```python
from build123d import *

# Parameters (mm, degrees)
ESQUISSE1_R             = 40
BOSS_EXTRU_1_DEPTH      = 78
ESQUISSE2_W             = 36.5
ESQUISSE2_H             = 3
ENL_V_MAT_EXTRU_1_DEPTH = 78
ESQUISSE3_R             = 3
ENL_V_MAT_EXTRU_2_DEPTH = 15


with BuildPart() as part:
    # Esquisse1 → Boss.-Extru.1 (new body)
    with BuildSketch(Plane.XY):
        with BuildLine():
            Line((-75, 0), (75, 0))
            Line((75, 0), (75, 15))
            Line((75, 15), (56.5, 15))
            Line((56.5, 15), (56.5, 83))
            Line((56.5, 83), (43.8178046, 83))
            ThreePointArc((43.8178046, 83), (0, 107), (-43.8178046, 83))
            Line((-43.8178046, 83), (-56.5, 83))
            Line((-56.5, 83), (-56.5, 15))
            Line((-56.5, 15), (-75, 15))
            Line((-75, 15), (-75, 0))
        make_face()
        with Locations((0, 55)):
            Circle(ESQUISSE1_R, mode=Mode.SUBTRACT)
    extrude(amount=BOSS_EXTRU_1_DEPTH)

    # Esquisse2 → Enlèv. mat.-Extru.1 (cut)
    with BuildSketch(Plane.XY.offset(78)):
        with Locations((38.25, 55)):
            Rectangle(ESQUISSE2_W, ESQUISSE2_H)
    extrude(amount=-ENL_V_MAT_EXTRU_1_DEPTH, mode=Mode.SUBTRACT)

    # Esquisse3 → Enlèv. mat.-Extru.2 (cut)
    with BuildSketch(Plane(origin=(0, 15, 0), x_dir=(1, 0, 0), z_dir=(0, 1, 0))):
        with Locations(Location((-65, -39, 0), (0, 0, 180))):
            Circle(ESQUISSE3_R)
        with Locations(Location((-65, -14, 0), (0, 0, 180))):
            Circle(ESQUISSE3_R)
        with Locations(Location((-65, -64, 0), (0, 0, 180))):
            Circle(ESQUISSE3_R)
        with Locations(Location((65, -64, 0), (0, 0, 180))):
            Circle(ESQUISSE3_R)
        with Locations(Location((65, -14, 0), (0, 0, 180))):
            Circle(ESQUISSE3_R)
        with Locations(Location((65, -39, 0), (0, 0, 180))):
            Circle(ESQUISSE3_R)
    extrude(amount=-ENL_V_MAT_EXTRU_2_DEPTH, mode=Mode.SUBTRACT)


solid = part.part
```
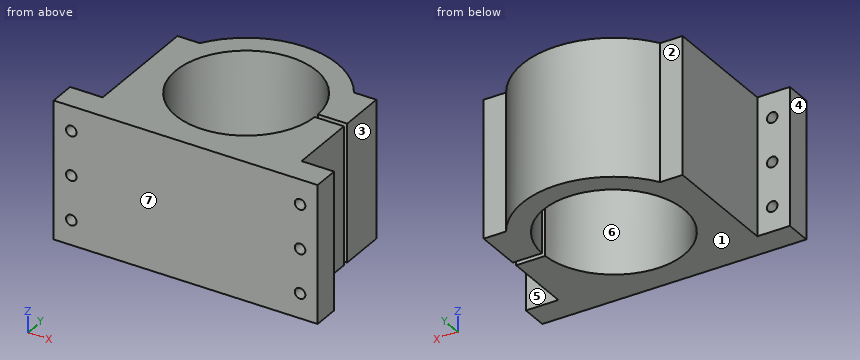
Geometry check sheet. Reference: the model listing, model coordinates, mm. Face numbers are marked on the shaded views. A direction names the side the tool comes from. Coordinates: 2 decimals unless noted, no trailing zeros. Write each loop counter-clockwise with the first axis right and the second up, starting at its lowest first coordinate (ties: lowest second). Pieces come first, ordered by that corner, then holes. Notation, with made-up numbers: M 1.5,35 L 38.5,35 A26 ccw 38.5,50 Z; hole C -13,8.5 d11. An arc over 180 degrees is marked long. Use one line per item in the form item = value. Start each with the question number.
1) Go/stop test with flat-tipped pins: pin 1 Ø9.5 at (x, z) = (-65, 14) entering from +Y; pin 2 Ø8 at (y, z) = (83.5, 34) entering from -X; pin 3 Ø20.5 at (x, z) = (66.5, 37) entering from +Y; pin 4 Ø5 at (x, z) = (65, 39) entering from +Y. Record where each tip stops, or that it passes through.
2) Thickness scan on probe 1 along Z at (x, y) = (65, 9); probe 2 along X at (y, z) = (12, 12); probe 3 along Y at (x, z) = (54, 8). Record the ranges inside material, lowest first. Write a range as from..to.
3) Set-up check for the marked faces 1, 2 and 3: record each of +Z, -Z, +X, -X, +Y, -Y from which the full face is reachable in a straight line by a thin tool's end or side.
4) Release check for a two-part mould opening along Y. For the marked faces 4, 5, 6 and 7 record: pulls with the +Y half, pulls with the -Y half, needs draft (parallel to the pull), parting line crosses it, or undercut.
5) Section check B-B on z = 39. Enter the section's corners in (x, y), and give its area (3 significant figures).
6) Section check D-D on x = -9. Enter the section's corners in (y, z).
7) Section check C-C on y = 75. Enter the section's corners in (x, z), and give its area (3 significant figures).
8) Section check A-A on x = 65. Enter the section's corners in (y, z), and give its area (3 significant figures).
Responses:
q1.pin_1 = 15
q1.pin_2 = -56.5
q1.pin_3 = 83
q1.pin_4 = through
q2.probe_1 = 0..11, 17..36, 42..61, 67..78
q2.probe_2 = -75..-67.24, -62.76..62.76, 67.24..75
q2.probe_3 = 0..53.5, 56.5..83
q3.face_1 = -Z, +X, -X, +Y, -Y
q3.face_2 = +Z, -Z, -X, +Y
q3.face_3 = +Z, -Z, +X, +Y
q4.face_4 = needs draft
q4.face_5 = pulls with the +Y half
q4.face_6 = undercut
q4.face_7 = pulls with the -Y half
q5.outline = M -75,0 L -68,0 L -68,15 L -75,15 Z; M -62,0 L 62,0 L 62,15 L 56.5,15 L 56.5,53.5 L 39.97,53.5 A40 cw long 39.97,56.5 L 56.5,56.5 L 56.5,83 L 43.82,83 A52 ccw -43.82,83 L -56.5,83 L -56.5,15 L -62,15 Z; M 68,0 L 75,0 L 75,15 L 68,15 Z
q5.area = 6,160 mm2
q6.outline = M 0,0 L 16.03,0 L 16.03,78 L 0,78 Z; M 93.97,0 L 106.22,0 L 106.22,78 L 93.97,78 Z
q7.outline = M -56.5,0 L -34.64,0 L -34.64,78 L -56.5,78 Z; M 34.64,0 L 56.5,0 L 56.5,78 L 34.64,78 Z
q7.area = 3,410 mm2
q8.outline = M 0,0 L 15,0 L 15,11 L 0,11 Z; M 0,17 L 15,17 L 15,36 L 0,36 Z; M 0,42 L 15,42 L 15,61 L 0,61 Z; M 0,67 L 15,67 L 15,78 L 0,78 Z
q8.area = 900 mm2
